Autodesk Fusion 360 part; units mm, degrees
sketch "Sketch1" plane through (0, 0, 0) normal (1, 0, 0) x (0, 0, -1)
sketch "Sketch2" plane through (0, 0, 0) normal (0, 1, 0) x (1, 0, 0)
  line L0 (0, 0) -> (50, 0)
  line L1 (50, 0) -> (50, 50)
  line L2 (50, 50) -> (0, 50)
  line L3 (0, 50) -> (0, 0)
  line L4 (-5, -5) -> (55, -5)
  line L5 (55, -5) -> (55, 55)
  line L6 (55, 55) -> (-5, 55)
  line L7 (-5, 55) -> (-5, -5)
  dimension "d1" = 50
  dimension "d2" = 50
  dimension "d3" = 5
extrude "Extrude1" add sketch "Sketch2" along normal blind 20
extrude "Extrude2" add sketch "Sketch2" along normal blind 5 contours L0 L1 L2 L3
sketch "Sketch3" plane through (-5, 0, 0) normal (-1, 0, 0) x (0, 0, 1)
  line L0 (-55, 0) -> (5, 0)
  line L1 (5, 0) -> (5, 20)
  line L2 (5, 20) -> (-55, 20)
  line L3 (-55, 20) -> (-55, 0)
  line L4 (-25, 20) -> (-25, 12.5) construction
  circle A0 centre (-25, 12.5) radius 2.5
  dimension "d8" = 7.5
  dimension "d9" = 5
extrude "Extrude3" cut sketch "Sketch3" against normal blind 163 contours A0
Geometry: final body of the model. Coordinates: model frame, mm. A direction names the side the tool comes from. Round coordinates to 2 decimals unless told otherwise and drop trailing zeros. Write each loop counter-clockwise with the first axis right and the second up, starting at its lowest first coordinate (ties: lowest second). Pieces come first, ordered by that corner, then holes.
Item 1: Section query A-A (y = 17.5). Return loops of the section in (x, z), plus the area to 3 significant figures.
Item 2: Mould query, pull axis Y, two halves, no side actions, for faces 3 (the face through (52.46, 10.06, -25.54)), 4 (the face through (-2.54, 10.06, -25.54)), 5 (the face through (-2, 20, -25)), 6 (the face through (0, 9, -25)). Classes: +Y half, -Y half, draft (parallel to the pull), parting line (faces both ways), or undercut.
Item 3: Section query D-D (x = 15.5). Return loops of the section in (y, z), plus the area to 3 significant figures.
Item 4: Section query B-B (z = -25). Return loops of the section in (x, y), plus the area to 3 significant figures.
Item 5: Pin query (flat end, axial travel): P1, Ø25, axis at x = 22.5, z = -25.5, coming from the +Y side. Return the tip coordinate at first contact, or that it passes through.
Item 6: Set-up query: faces 1 (the face through (25, 12, -50)), 2 (the face through (25, 0, -25)). Return all of +Z, -Z, +X, -X, +Y, -Y with unobstructed straight access to the full face (end or side cutting, diameter ignored); none if empty.
Item 7: Section query C-C (y = 12.5). Return loops of the section in (x, z).
Item 8: Material intervals for L1, parallel to Y at x = 52.85, z = -25; L2, parallel to Z at x = 24, y = 13.25; L3, parallel to X at y = 7.5, z = -14.5, sorted ascending.
Completed:
1. outline: (-5, -55) - (55, -55) - (55, 5) - (-5, 5) - close; hole (0, -50) - (50, -50) - (50, 0) - (0, 0) - close
1. area: 1,100 mm2
2. face 3: undercut
2. face 4: undercut
2. face 5: +Y half
2. face 6: draft
3. outline: (0, -55) - (20, -55) - (20, -50) - (5, -50) - (5, 0) - (20, 0) - (20, 5) - (0, 5) - close
3. area: 450 mm2
4. outline: (-5, 0) - (55, 0) - (55, 10) - (50, 10) - (50, 5) - (0, 5) - (0, 10) - (-5, 10) - close; (-5, 15) - (0, 15) - (0, 20) - (-5, 20) - close; (50, 15) - (55, 15) - (55, 20) - (50, 20) - close
4. area: 400 mm2
5. P1: stops at y = 5
6. face 1: +Y
6. face 2: +Z, -Z, +X, -X, -Y
7. outline: (-5, -55) - (55, -55) - (55, -27.5) - (50, -27.5) - (50, -50) - (0, -50) - (0, -27.5) - (-5, -27.5) - close; (-5, -22.5) - (0, -22.5) - (0, 0) - (50, 0) - (50, -22.5) - (55, -22.5) - (55, 5) - (-5, 5) - close
8. L1: y = 0 to 10, 15 to 20
8. L2: z = -55 to -50, 0 to 5
8. L3: x = -5 to 0, 50 to 55
